Work out the finished part from the listing and answer in its coordinate system (mm). Give positions to 0.01 mm unless a question says otherwise; leave off trailing zeros. Loops run counter-clockwise (first coordinate to the right, second up) from the corner with the lowest first, then second, coordinate; pieces in that order, holes last. Notation, with made-up numbers: (10, -27.5) -> (27, -27.5) arc R35 ccw to (27, 5.5) -> close; hole circle Ø1 at (-22.5, -5). An arc over 180 degrees is marked (long way). Answer as CSV lines item,"result". Start each with the question number.
1. Find section B-B, the plane x = 136. Give the vertices of the cut face in (y, z) (3 decimals), and give its area (4 significant figures).
2. Find section C-C, the plane z = -76. Give the vertices of the cut face in (x, y) (3 decimals), and give its area (3 significant figures).
3. Find section A-A, the plane y = 1.4. Give the vertices of the cut face in (x, z).
4. Determine the mould class of faces 1 (the face through (202.02, 1.57, -72.73)), 2 (the face through (170, 0, -41)), 3 (the face through (227.72, 1.565, -122.255)), 4 (the face through (187, 1.6, -72.4)) for opening direction X: +X half, -X half, draft (parallel to the pull), parting line (faces both ways), or undercut.
5. Flat-ended cylindrical pins translate along their axes: pin 1 Ø2.5 at (x, z) = (5.25, -5) entering from +Y; pin 2 Ø1.6 at (y, z) = (1.5, -32.5) entering from +X; pin 3 Ø1 at (y, z) = (1.5, -34) entering from -X; pin 4 Ø1 at (y, z) = (2.5, -75) entering from -X. Find the tip coordinate at first contact, or state that the pin passes through.
6. Find the intervals of material crossed by line 1 along X through (y, z) = (2.05, -5); line 2 along Z through (x, y) = (146, 1.05); line 3 along X through (y, z) = (3.05, -104), in increasing order.
from build123d import *

# Parameters (mm, degrees)
SKETCH1_R           = 1.4605
SKETCH1_R_2         = 12.7
BOSS_EXTRUDE1_DEPTH = 3.175
FILLET1_R           = 2.921


with BuildPart() as part:
    # Sketch1 → Boss-Extrude1 (new body)
    with BuildSketch(Plane(origin=(0, 0, 0), x_dir=(1, 0, 0), z_dir=(0, 1, 0))):
        with BuildLine():
            Line((0, 0), (172.7, 0))
            Line((172.7, 0), (172.7, 45.39))
            Line((172.7, 45.39), (231.20829613, 99.949868805))
            ThreePointArc((231.20829613, 99.949868805), (215.791893749, 130.275875463), (212.732452536, 96.394140536))
            Line((212.732452536, 96.394140536), (162.7, 49.73812375))
            Line((162.7, 49.73812375), (162.7, 10))
            Line((162.7, 10), (0, 10))
            Line((0, 10), (0, 0))
        make_face()
        with Locations(Location((5.25, 5, 0), (0, 0, 270))):
            Circle(SKETCH1_R, mode=Mode.SUBTRACT)
        with Locations(Location((167.45, 5, 0), (0, 0, 270))):
            Circle(SKETCH1_R, mode=Mode.SUBTRACT)
        with Locations(Location((219.136925156, 112.894829324, 0), (0, 0, 270))):
            Circle(SKETCH1_R_2, mode=Mode.SUBTRACT)
    extrude(amount=BOSS_EXTRUDE1_DEPTH)

    # Fillet1
    fillet1_edges = [part.edges().sort_by_distance(p)[0] for p in [
        (0, 1.5875, -10),
        (162.7, 1.5875, -10),
        (162.7, 1.5875, -49.73812375),
        (212.732452536, 1.5875, -96.394140536),
        (172.7, 1.5875, -45.39),
        (172.7, 1.5875, 0),
        (0, 1.5875, 0),
    ]]
    fillet(fillet1_edges, radius=FILLET1_R)


solid = part.part
Resolved:
1,outline,"(0, -10) -> (3.175, -10) -> (3.175, 0) -> (0, 0) -> close"
1,area,"31.75 mm^2"
2,outline,"(190.862, 0) -> (205.525, 0) -> (205.525, 3.175) -> (190.862, 3.175) -> close"
2,area,"46.6 mm^2"
3,outline,"(0, -7.08) arc R2.92 ccw to (2.92, -10) -> (159.78, -10) arc R2.92 cw to (162.7, -12.92) -> (162.7, -48.47) arc R2.92 ccw to (163.63, -50.6) -> (209.72, -93.58) arc R2.92 cw to (209.34, -98.15) arc R17.7 ccw (long way) to (231.21, -99.95) -> (173.63, -46.26) arc R2.92 cw to (172.7, -44.12) -> (172.7, -2.92) arc R2.92 ccw to (169.78, 0) -> (2.92, 0) arc R2.92 ccw to (0, -2.92) -> close; hole circle Ø2.92 at (5.25, -5); hole circle Ø2.92 at (167.45, -5); hole circle Ø25.4 at (219.14, -112.89)"
4,face 1,"+X half"
4,face 2,"draft"
4,face 3,"undercut"
4,face 4,"-X half"
5,pin 1,"passes through"
5,pin 2,"stops at x = 172.7"
5,pin 3,"stops at x = 162.7"
5,pin 4,"stops at x = 189.25"
6,line 1,"x = 0 to 3.79, 6.71 to 165.99, 168.91 to 172.7"
6,line 2,"z = -10 to 0"
6,line 3,"x = 203.83 to 210.07, 228.2 to 234.44"
